Read the model definition and answer for the solid it produces. Units are mm, in the model's axes. Coordinates: 2 decimals unless noted, no trailing zeros. Write each loop counter-clockwise with the first axis right and the second up, starting at its lowest first coordinate (ties: lowest second). Pieces come first, ordered by that corner, then holes. Notation, with made-up numbers: (-4.75, 28.5) -> (29.25, 28.5) arc R36 cw to (29.25, 64.5) -> close; hole circle Ø11 at (23, 66). An arc over 180 degrees is marked (long way). Answer as a JSON object with one key per item and string values. Group by question number.
(1) Find section B-B (x = -189.5). Give the vertices of the cut face in (y, z) (3 decimals).
(2) For a pull along Z with two mould halves and no side action, classify faces 1 (the face through (-4, 13, -3.175)), 2 (the face through (-4, 13, 3.175)) as +Z half, -Z half, draft (parallel to the pull), parting line (faces both ways), or undercut.
(3) Straight lines are drawn through the part: L1, parallel to Y at x = 193.5, z = 0; L2, parallel to Y at x = -19, z = 3; L3, parallel to X at y = -1, z = -1 (3 decimals). For each, find the intervals that lie inside material, in ascending order.
(4) Flat-ended cylindrical pins translate along their axes: P1, Ø3, axis at x = 80.5, z = -1.5, coming from the -Y side; P2, Ø8, axis at x = -67, y = -1, coming from the -Z side (3 decimals); P3, Ø1.5, axis at y = -2.5, z = 0.5, coming from the +X side. Find the tip coordinate at first contact, or state that the pin passes through.
(5) Find section A-A (y = 18). Count the separate pieces of the cut face and the enclosed holes in it, then the cut area to 3 significant figures.
from build123d import *

# Parameters (mm, degrees)
SKETCH1_W           = 571.5
SKETCH1_H           = 6.35
BOSS_EXTRUDE1_DEPTH = 25.4
BOSS_EXTRUDE2_DEPTH = 6.35
CUT_EXTRUDE1_DEPTH  = 287.946937603


with BuildPart() as part:
    # Sketch1 → Boss-Extrude1 (new body)
    with BuildSketch(Plane(origin=(0, 0, 0), x_dir=(1, 0, 0), z_dir=(0, 1, 0))):
        Rectangle(SKETCH1_W, SKETCH1_H)
    extrude(amount=BOSS_EXTRUDE1_DEPTH)

    # Sketch2 → Boss-Extrude2 (add)
    with BuildSketch(Plane.XZ):
        with BuildLine():
            Line((-273.05, 2.54), (-273.05, -2.54))
            ThreePointArc((-273.05, -2.54), (-275.59, 0), (-273.05, 2.54))
        make_face()
        with BuildLine():
            Line((-136.525, 2.54), (-136.525, -2.54))
            ThreePointArc((-136.525, -2.54), (-139.065, 0), (-136.525, 2.54))
        make_face()
        with BuildLine():
            Line((0, 2.54), (0, -2.54))
            ThreePointArc((0, -2.54), (-2.54, 0), (0, 2.54))
        make_face()
        with BuildLine():
            Line((136.525, 2.54), (136.525, -2.54))
            ThreePointArc((136.525, -2.54), (133.985, 0), (136.525, 2.54))
        make_face()
        with BuildLine():
            Line((273.05, 2.54), (273.05, -2.54))
            ThreePointArc((273.05, -2.54), (270.51, 0), (273.05, 2.54))
        make_face()
    extrude(amount=BOSS_EXTRUDE2_DEPTH)

    # Sketch3 → Cut-Extrude1 (cut, through all)
    with BuildSketch(Plane.XY.offset(3.175)):
        with BuildLine():
            Line((-246.38, 38.1), (-246.38, 12.7))
            ThreePointArc((-246.38, 12.7), (-248.92, 10.16), (-251.46, 12.7))
            Line((-251.46, 12.7), (-251.46, 38.1))
            ThreePointArc((-251.46, 38.1), (-248.92, 40.64), (-246.38, 38.1))
        make_face()
        with BuildLine():
            Line((-209.55, 38.1), (-209.55, 12.7))
            ThreePointArc((-209.55, 12.7), (-212.09, 10.16), (-214.63, 12.7))
            Line((-214.63, 12.7), (-214.63, 38.1))
            ThreePointArc((-214.63, 38.1), (-212.09, 40.64), (-209.55, 38.1))
        make_face()
        with BuildLine():
            Line((-172.72, 38.1), (-172.72, 12.7))
            ThreePointArc((-172.72, 12.7), (-175.26, 10.16), (-177.8, 12.7))
            Line((-177.8, 12.7), (-177.8, 38.1))
            ThreePointArc((-177.8, 38.1), (-175.26, 40.64), (-172.72, 38.1))
        make_face()
        with BuildLine():
            Line((-135.89, 38.1), (-135.89, 12.7))
            ThreePointArc((-135.89, 12.7), (-138.43, 10.16), (-140.97, 12.7))
            Line((-140.97, 12.7), (-140.97, 38.1))
            ThreePointArc((-140.97, 38.1), (-138.43, 40.64), (-135.89, 38.1))
        make_face()
        with BuildLine():
            Line((-99.06, 38.1), (-99.06, 12.7))
            ThreePointArc((-99.06, 12.7), (-101.6, 10.16), (-104.14, 12.7))
            Line((-104.14, 12.7), (-104.14, 38.1))
            ThreePointArc((-104.14, 38.1), (-101.6, 40.64), (-99.06, 38.1))
        make_face()
        with BuildLine():
            Line((-62.23, 38.1), (-62.23, 12.7))
            ThreePointArc((-62.23, 12.7), (-64.77, 10.16), (-67.31, 12.7))
            Line((-67.31, 12.7), (-67.31, 38.1))
            ThreePointArc((-67.31, 38.1), (-64.77, 40.64), (-62.23, 38.1))
        make_face()
        with BuildLine():
            Line((-25.4, 38.1), (-25.4, 12.7))
            ThreePointArc((-25.4, 12.7), (-27.94, 10.16), (-30.48, 12.7))
            Line((-30.48, 12.7), (-30.48, 38.1))
            ThreePointArc((-30.48, 38.1), (-27.94, 40.64), (-25.4, 38.1))
        make_face()
        with BuildLine():
            Line((11.43, 38.1), (11.43, 12.7))
            ThreePointArc((11.43, 12.7), (8.89, 10.16), (6.35, 12.7))
            Line((6.35, 12.7), (6.35, 38.1))
            ThreePointArc((6.35, 38.1), (8.89, 40.64), (11.43, 38.1))
        make_face()
        with BuildLine():
            Line((48.26, 38.1), (48.26, 12.7))
            ThreePointArc((48.26, 12.7), (45.72, 10.16), (43.18, 12.7))
            Line((43.18, 12.7), (43.18, 38.1))
            ThreePointArc((43.18, 38.1), (45.72, 40.64), (48.26, 38.1))
        make_face()
        with BuildLine():
            Line((85.09, 38.1), (85.09, 12.7))
            ThreePointArc((85.09, 12.7), (82.55, 10.16), (80.01, 12.7))
            Line((80.01, 12.7), (80.01, 38.1))
            ThreePointArc((80.01, 38.1), (82.55, 40.64), (85.09, 38.1))
        make_face()
        with BuildLine():
            Line((121.92, 38.1), (121.92, 12.7))
            ThreePointArc((121.92, 12.7), (119.38, 10.16), (116.84, 12.7))
            Line((116.84, 12.7), (116.84, 38.1))
            ThreePointArc((116.84, 38.1), (119.38, 40.64), (121.92, 38.1))
        make_face()
        with BuildLine():
            Line((158.75, 38.1), (158.75, 12.7))
            ThreePointArc((158.75, 12.7), (156.21, 10.16), (153.67, 12.7))
            Line((153.67, 12.7), (153.67, 38.1))
            ThreePointArc((153.67, 38.1), (156.21, 40.64), (158.75, 38.1))
        make_face()
        with BuildLine():
            Line((195.58, 38.1), (195.58, 12.7))
            ThreePointArc((195.58, 12.7), (193.04, 10.16), (190.5, 12.7))
            Line((190.5, 12.7), (190.5, 38.1))
            ThreePointArc((190.5, 38.1), (193.04, 40.64), (195.58, 38.1))
        make_face()
        with BuildLine():
            Line((232.41, 38.1), (232.41, 12.7))
            ThreePointArc((232.41, 12.7), (229.87, 10.16), (227.33, 12.7))
            Line((227.33, 12.7), (227.33, 38.1))
            ThreePointArc((227.33, 38.1), (229.87, 40.64), (232.41, 38.1))
        make_face()
        with BuildLine():
            Line((269.24, 38.1), (269.24, 12.7))
            ThreePointArc((269.24, 12.7), (266.7, 10.16), (264.16, 12.7))
            Line((264.16, 12.7), (264.16, 38.1))
            ThreePointArc((264.16, 38.1), (266.7, 40.64), (269.24, 38.1))
        make_face()
    extrude(amount=-CUT_EXTRUDE1_DEPTH, mode=Mode.SUBTRACT)


solid = part.part
Results below:
{
 "1": {"outline": "(0, -3.175) -> (25.4, -3.175) -> (25.4, 3.175) -> (0, 3.175) -> close"},
 "2": {"face 1": "-Z half", "face 2": "+Z half"},
 "3": {"L1": "y = 0 to 10.2", "L2": "y = 0 to 25.4", "L3": "x = -275.385 to -273.05, -138.86 to -136.525, -2.335 to 0, 134.19 to 136.525, 270.715 to 273.05"},
 "4": {"P1": "stops at y = 0", "P2": "stops at z = -3.175", "P3": "stops at x = 273.05"},
 "5": {"separate pieces": "16", "enclosed holes": "0", "area": "3,150 mm2"}
}
